```python
from build123d import *

# Parameters (mm, degrees)
SKETCH1_W   = 1.5
SKETCH1_H   = 7
SKETCH1_W_2 = 4
SKETCH1_H_2 = 6


with BuildPart() as part:
    # Sketch1 → Revolve1 (revolve)
    with BuildSketch(Plane.XY):
        with Locations((-10.25, 0)):
            Rectangle(SKETCH1_W, SKETCH1_H)
        with Locations((-7.5, 0)):
            Rectangle(SKETCH1_W_2, SKETCH1_H_2)
        with Locations((-4.75, 0)):
            Rectangle(SKETCH1_W, SKETCH1_H)
    revolve(axis=Axis((0, -3.362712124, 0), (0, 1, 0)))


solid = part.part
```
Can you work these out from the model? Positions are in its coordinate system, mm. A direction names the side the tool comes from. Round coordinates to 2 decimals unless told otherwise and drop trailing zeros. Loops run counter-clockwise (first coordinate to the right, second up) from the corner with the lowest first, then second, coordinate; pieces in that order, holes last. Notation, with made-up numbers: (87, 28) -> (138, 28) arc R10 cw to (138, 33) -> close; hole circle Ø4 at (55, -35). An arc over 180 degrees is marked (long way). One line per item, written item: value. Start each with the question number.
1. If we section it at B-B, the plane x = 0: Write out the boundary of the cut face in (y, z).
2. For pin 1 (6.5 mm diameter, centred on x = 0, z = 0, fed in from +Y); pin 2 (1 mm diameter, centred on x = -5.5, y = -1.5, fed in from -Z); pin 3 (1.5 mm diameter, centred on y = -2.5, z = 5.5, fed in from -X), each with a flat end and sliding along its axis, tell me the tip position at first contact or that it passes through.
3. If we section it at A-A, the plane z = 0: Write out the boundary of the cut face in (x, y), then the cut area to 3 significant figures.
4. If we section it at C-C, the plane z = 4.5: Write out the boundary of the cut face in (x, y).
5. If I drill on probe 1 along Z at (x, y) = (0, -3.4); probe 2 along Z at (x, y) = (0, 2.75); probe 3 along Y at (x, z) = (5, -8), over which ranges is the centre line in solid material (lowest first)?
6. If we mould it in two halves opening along X, with no side actions, what happens to faces 4 (the cylindrical face through (2.38, 0.05, -10.74)), 5 (the cylindrical face through (-4.38, -3.25, -8.43)), 6 (the flat face through (4, 3.5, -2))? For each: pulls with the +X half, pulls with the -X half, needs draft (parallel to the pull), parting line crosses it, or undercut.
7. For faces 1 (the cylindrical face through (1.19, -3.25, -5.37)), 2 (the cylindrical face through (-4.38, 3.25, -8.43)), 3 (the cylindrical face through (0.867, 0.049, -3.905)), which set-ups out of +Z, -Z, +X, -X, +Y, -Y let a thin tool reach every point of the face, with its end or its side?
8. If we section it at D-D, the plane y = 1: Write out the boundary of the cut face in (x, z), then the cut area to 3 significant figures.
Calculated:
1. outline: (-3.5, -11) -> (3.5, -11) -> (3.5, -9.5) -> (3, -9.5) -> (3, -5.5) -> (3.5, -5.5) -> (3.5, -4) -> (-3.5, -4) -> (-3.5, -5.5) -> (-3, -5.5) -> (-3, -9.5) -> (-3.5, -9.5) -> close; (-3.5, 4) -> (3.5, 4) -> (3.5, 5.5) -> (3, 5.5) -> (3, 9.5) -> (3.5, 9.5) -> (3.5, 11) -> (-3.5, 11) -> (-3.5, 9.5) -> (-3, 9.5) -> (-3, 5.5) -> (-3.5, 5.5) -> close
2. pin 1: passes through
2. pin 2: stops at z = -9.8
2. pin 3: stops at x = -9.92
3. outline: (-11, -3.5) -> (-9.5, -3.5) -> (-9.5, -3) -> (-5.5, -3) -> (-5.5, -3.5) -> (-4, -3.5) -> (-4, 3.5) -> (-5.5, 3.5) -> (-5.5, 3) -> (-9.5, 3) -> (-9.5, 3.5) -> (-11, 3.5) -> close; (4, -3.5) -> (5.5, -3.5) -> (5.5, -3) -> (9.5, -3) -> (9.5, -3.5) -> (11, -3.5) -> (11, 3.5) -> (9.5, 3.5) -> (9.5, 3) -> (5.5, 3) -> (5.5, 3.5) -> (4, 3.5) -> close
3. area: 90.0 mm²
4. outline: (-10.04, -3.5) -> (-8.37, -3.5) -> (-8.37, -3) -> (-3.16, -3) -> (-3.16, -3.5) -> (3.16, -3.5) -> (3.16, -3) -> (8.37, -3) -> (8.37, -3.5) -> (10.04, -3.5) -> (10.04, 3.5) -> (8.37, 3.5) -> (8.37, 3) -> (3.16, 3) -> (3.16, 3.5) -> (-3.16, 3.5) -> (-3.16, 3) -> (-8.37, 3) -> (-8.37, 3.5) -> (-10.04, 3.5) -> close
5. probe 1: z = -11 to -9.5, -5.5 to -4, 4 to 5.5, 9.5 to 11
5. probe 2: z = -11 to -4, 4 to 11
5. probe 3: y = -3 to 3
6. face 4: parting line crosses it
6. face 5: undercut
6. face 6: needs draft
7. face 1: -Y
7. face 2: +Y
7. face 3: +Y, -Y
8. outline: circle Ø22 at (0, 0); hole circle Ø8 at (0, 0)
8. area: 330 mm²
